```python
from build123d import *

# Parameters (mm, degrees)
BOX008_W                = 10
BOX008_H                = 2.6
BOX008_DEPTH            = 2.6
CYLINDER004_R           = 6
CYLINDER004_DEPTH       = 10
CYLINDER004_PITCH_ANGLE = 90
CYLINDER005_R           = 3.8
CYLINDER005_DEPTH       = 10
CYLINDER005_PITCH_ANGLE = 90
BOX006_W                = 10
BOX006_H                = 14.5
BOX006_DEPTH            = 8.9
BOX007_W                = 5.1
BOX007_H                = 22.8
BOX007_DEPTH            = 18
CYLINDER001_R           = 1
CYLINDER001_DEPTH       = 8
BOX003_W                = 5.1
BOX003_H                = 5.1
BOX003_DEPTH            = 23
CYLINDER003_R           = 1
CYLINDER003_DEPTH       = 8
BOX005_W                = 5.1
BOX005_H                = 5.1
BOX005_DEPTH            = 23
CYLINDER002_R           = 1
CYLINDER002_DEPTH       = 8
BOX004_W                = 5.1
BOX004_H                = 5.1
BOX004_DEPTH            = 23
CYLINDER_R              = 1
CYLINDER_DEPTH          = 8
BOX002_W                = 5.1
BOX002_H                = 5.1
BOX002_DEPTH            = 23
BOX001_W                = 29.8
BOX001_H                = 29.8
BOX001_DEPTH            = 23
BOX_W                   = 33
BOX_H                   = 33
BOX_DEPTH               = 23
FILLET_R                = 2.5


with BuildPart() as obj1:
    # Box008 → Box008 (new body)
    with BuildSketch(Plane(origin=(51, 19, 1.6), x_dir=(1, 0, 0), z_dir=(0, 0, 1))):
        with Locations((5, 1.3)):
            Rectangle(BOX008_W, BOX008_H)
    extrude(amount=BOX008_DEPTH)


with BuildPart() as aviator:
    # Cylinder004 → Cylinder004 (new body)
    with BuildSketch(Plane.XY):
        Circle(CYLINDER004_R)
    extrude(amount=CYLINDER004_DEPTH)


with BuildPart() as aviator_1:
    # Cylinder004 pitch: moved
    add(aviator.part.rotate(Axis((0, 0, 0), (0, 1, 0)), CYLINDER004_PITCH_ANGLE))


with BuildPart() as aviator_2:
    # Cylinder004 placement: moved
    add(aviator_1.part.moved(Location((50, 11, 11))))


with BuildPart() as obj2:
    # Cylinder005 → Cylinder005 (new body)
    with BuildSketch(Plane.XY):
        Circle(CYLINDER005_R)
    extrude(amount=CYLINDER005_DEPTH)


with BuildPart() as obj2_1:
    # Cylinder005 pitch: moved
    add(obj2.part.rotate(Axis((0, 0, 0), (0, 1, 0)), CYLINDER005_PITCH_ANGLE))


with BuildPart() as obj2_2:
    # Cylinder005 placement: moved
    add(obj2_1.part.moved(Location((50, 25, 11))))


with BuildPart() as obj3:
    # Box006 → Box006 (new body)
    with BuildSketch(Plane(origin=(22.5, 9.25, 7.5), x_dir=(1, 0, 0), z_dir=(0, 0, 1))):
        with Locations((5, 7.25)):
            Rectangle(BOX006_W, BOX006_H)
    extrude(amount=BOX006_DEPTH)

    # Fusion003: union Aviator, obj2
    add(aviator_2.part)
    add(obj2_2.part)


with BuildPart() as obj4:
    # Box007 → Box007 (new body)
    with BuildSketch(Plane(origin=(53.4, 5.1, 0), x_dir=(1, 0, 0), z_dir=(0, 0, 1))):
        with Locations((2.55, 11.4)):
            Rectangle(BOX007_W, BOX007_H)
    extrude(amount=BOX007_DEPTH)


with BuildPart() as obj5:
    # Cylinder001 → Cylinder001 (new body)
    with BuildSketch(Plane(origin=(2.55, 2.55, 15), x_dir=(1, 0, 0), z_dir=(0, 0, 1))):
        Circle(CYLINDER001_R)
    extrude(amount=CYLINDER001_DEPTH)


with BuildPart() as obj6:
    # Box003 → Box003 (new body)
    with BuildSketch(Plane.XY):
        with Locations((2.55, 2.55)):
            Rectangle(BOX003_W, BOX003_H)
    extrude(amount=BOX003_DEPTH)

    # Cut002: cut obj5
    add(obj5.part, mode=Mode.SUBTRACT)


with BuildPart() as obj6_1:
    # Cut002 placement: moved
    add(obj6.part.moved(Location((53.4, 0, 0))))


with BuildPart() as obj7:
    # Cylinder003 → Cylinder003 (new body)
    with BuildSketch(Plane(origin=(2.55, 2.55, 15), x_dir=(1, 0, 0), z_dir=(0, 0, 1))):
        Circle(CYLINDER003_R)
    extrude(amount=CYLINDER003_DEPTH)


with BuildPart() as obj8:
    # Box005 → Box005 (new body)
    with BuildSketch(Plane.XY):
        with Locations((2.55, 2.55)):
            Rectangle(BOX005_W, BOX005_H)
    extrude(amount=BOX005_DEPTH)

    # Cut004: cut obj7
    add(obj7.part, mode=Mode.SUBTRACT)


with BuildPart() as obj8_1:
    # Cut004 placement: moved
    add(obj8.part.moved(Location((53.4, 27.9, 0))))


with BuildPart() as obj9:
    # Cylinder002 → Cylinder002 (new body)
    with BuildSketch(Plane(origin=(2.55, 2.55, 15), x_dir=(1, 0, 0), z_dir=(0, 0, 1))):
        Circle(CYLINDER002_R)
    extrude(amount=CYLINDER002_DEPTH)


with BuildPart() as obj10:
    # Box004 → Box004 (new body)
    with BuildSketch(Plane.XY):
        with Locations((2.55, 2.55)):
            Rectangle(BOX004_W, BOX004_H)
    extrude(amount=BOX004_DEPTH)

    # Cut003: cut obj9
    add(obj9.part, mode=Mode.SUBTRACT)


with BuildPart() as obj10_1:
    # Cut003 placement: moved
    add(obj10.part.moved(Location((25.5, 27.9, 0))))


with BuildPart() as obj11:
    # Cylinder → Cylinder (new body)
    with BuildSketch(Plane(origin=(2.55, 2.55, 15), x_dir=(1, 0, 0), z_dir=(0, 0, 1))):
        Circle(CYLINDER_R)
    extrude(amount=CYLINDER_DEPTH)


with BuildPart() as obj12:
    # Box002 → Box002 (new body)
    with BuildSketch(Plane.XY):
        with Locations((2.55, 2.55)):
            Rectangle(BOX002_W, BOX002_H)
    extrude(amount=BOX002_DEPTH)

    # Cut001: cut obj11
    add(obj11.part, mode=Mode.SUBTRACT)


with BuildPart() as obj12_1:
    # Cut001 placement: moved
    add(obj12.part.moved(Location((25.5, 0, 0))))

    # Fusion: union obj6, obj8, obj10
    add(obj6_1.part)
    add(obj8_1.part)
    add(obj10_1.part)


with BuildPart() as innen:
    # Box001 → Box001 (new body)
    with BuildSketch(Plane(origin=(1.6, 1.6, 1.6), x_dir=(1, 0, 0), z_dir=(0, 0, 1))):
        with Locations((14.9, 14.9)):
            Rectangle(BOX001_W, BOX001_H)
    extrude(amount=BOX001_DEPTH)


with BuildPart() as cut006:
    # Box → Box (new body)
    with BuildSketch(Plane.XY):
        with Locations((16.5, 16.5)):
            Rectangle(BOX_W, BOX_H)
    extrude(amount=BOX_DEPTH)

    # Cut: cut Innen
    add(innen.part, mode=Mode.SUBTRACT)


with BuildPart() as cut006_1:
    # Cut placement: moved
    add(cut006.part.moved(Location((25.5, 0, 0))))

    # Fusion001: union obj12
    add(obj12_1.part)

    # Fusion002: union obj4
    add(obj4.part)

    # Fillet
    fillet_edges = [cut006_1.edges().sort_by_distance(p)[0] for p in [
        (25.5, 0, 11.5),
        (25.5, 33, 11.5),
        (58.5, 0, 11.5),
        (30.6, 5.1, 12.3),
        (58.5, 33, 11.5),
        (30.6, 27.9, 12.3),
    ]]
    fillet(fillet_edges, radius=FILLET_R)

    # Cut005: cut obj3
    add(obj3.part, mode=Mode.SUBTRACT)

    # Cut006: cut obj1
    add(obj1.part, mode=Mode.SUBTRACT)


solid = cut006_1.part
```
Model file for the job. Use its own axes, mm. A direction names the side the tool comes from. Give positions to 0.01 mm unless a question says otherwise; leave off trailing zeros. Order: outer loops, then holes, each group sorted by start corner. A loop starts at its lowest first (then second) coordinate and runs counter-clockwise, first axis right, second up.
1) Saw through at C-C, the plane y = 17.5. Write the cut outline in (x, z), then the cut area to 3 significant figures.
2) Pin check, flat tips, straight feed: pin 1 (0.8 mm diameter, centred on x = 56.5, z = 3, fed in from +Y); pin 2 (0.6 mm diameter, centred on x = 55.5, y = 30, fed in from +Z). Stop position of each tip, or through.
3) Saw through at B-B, the plane y = 11. Write the cut outline in (x, z).
4) Mould opens along X. For faces 5 (the flat face through (26, 17, 7.5)), 6 (the cylindrical face through (26, 32, 12)), 7 (the flat face through (56.9, 16, 20)) say: +X half, -X half, draft (parallel to the pull), parting line (faces both ways), or undercut.
5) Saw through at D-D, the plane x = 35.5. Write the cut outline in (y, z).
6) Saw through at A-A, the plane x = 54.5. Write the cut outline in (y, z).
7) 3-axis set-ups, long thin cutter, end or side, ignore diameter. For faces 1 (the flat face through (26, 17, 16.4)), 2 (the flat face through (28, 30, 15)), 3 (the flat face through (42, 1, 23)), 4 (the flat face through (56, 19, 3)): which of +Z, -Z, +X, -X, +Y, -Y reach the whole face in a straight line?
8) Wall check: probe 1 along X at (y, z) = (2.55, 19); probe 2 along Y at (x, z) = (28.05, 19.75); probe 3 along Y at (x, z) = (54.9, 11). Give the ranges that are in metal, low to high.
Computed:
1. outline: (25.5, 0) - (58.5, 0) - (58.5, 23) - (56.9, 23) - (56.9, 18) - (53.4, 18) - (53.4, 1.6) - (27.1, 1.6) - (27.1, 7.5) - (25.5, 7.5) - close; (25.5, 16.4) - (27.1, 16.4) - (27.1, 23) - (25.5, 23) - close
1. area: 164 mm2
2. pin 1: stops at y = 33
2. pin 2: stops at z = 15
3. outline: (25.5, 0) - (58.5, 0) - (58.5, 5) - (53.4, 5) - (53.4, 1.6) - (27.1, 1.6) - (27.1, 7.5) - (25.5, 7.5) - close; (25.5, 16.4) - (27.1, 16.4) - (27.1, 23) - (25.5, 23) - close; (53.4, 17) - (58.5, 17) - (58.5, 23) - (56.9, 23) - (56.9, 18) - (53.4, 18) - close
4. face 5: draft
4. face 6: -X half
4. face 7: undercut
5. outline: (0, 0) - (33, 0) - (33, 23) - (31.4, 23) - (31.4, 1.6) - (1.6, 1.6) - (1.6, 23) - (0, 23) - close
6. outline: (0, 0) - (33, 0) - (33, 23) - (27.9, 23) - (27.9, 18) - (5.1, 18) - (5.1, 23) - (0, 23) - close; hole circle Ø12 at (11, 11); hole (19, 1.6) - (21.6, 1.6) - (21.6, 4.2) - (19, 4.2) - close; hole circle Ø7.6 at (25, 11)
7. face 1: -X
7. face 2: +Z
7. face 3: +Z, +X, -X, +Y, -Y
7. face 4: +X
8. probe 1: x = 25.5 to 27.1, 29.05 to 30.6, 53.4 to 54.95, 56.9 to 58.5
8. probe 2: y = 0 to 1.6, 3.55 to 5.1, 27.9 to 29.45, 31.4 to 33
8. probe 3: y = 0 to 5, 17 to 21.2, 28.8 to 33
